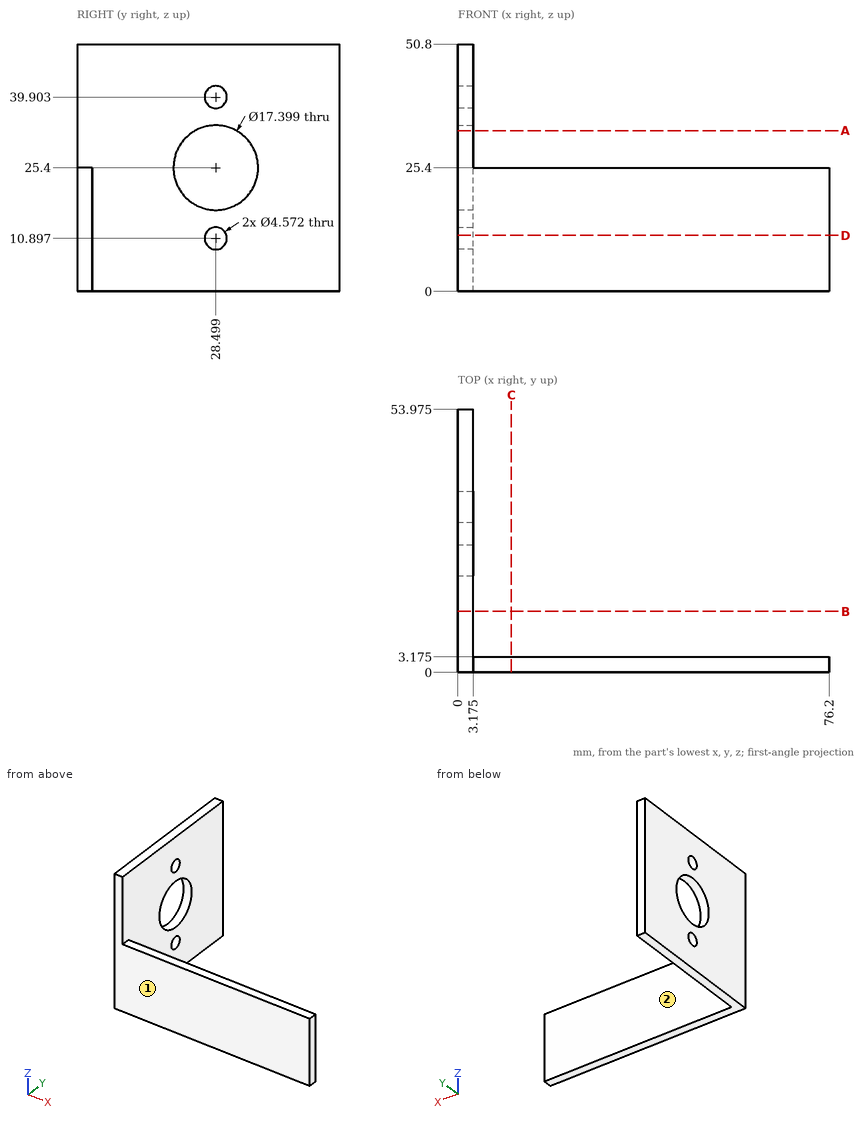
The drawing under review shows one solid part. Ordinate dimensions are in mm from its lowest x, y, z. A direction names the side the tool comes from. Coordinates: 2 decimals unless noted, no trailing zeros. Loops run counter-clockwise (first coordinate to the right, second up) from the corner with the lowest first, then second, coordinate; pieces in that order, holes last. Notation, with made-up numbers: (37.25, 64) - (55.25, 64) arc R12 ccw to (55.25, 80) - close; hole circle Ø1 at (46, -33.5). An arc over 180 degrees is marked (long way). Use CSV: the item, a comma, the result in double quotes. Start each with the question number.
1. To check wall thickness, follow probe 1 along Y at (x, z) = (0.85, 25.4) (1 decimal); probe 2 along X at (y, z) = (4, 5.5) (1 decimal). State the ranges of each line that lie inside material, in increasing order.
2. For the marked faces 1 and 2, list the 3-axis set-ups (+Z, -Z, +X, -X, +Y, -Y) from which the entire face can be reached by the end or side of a thin tool; tool diameter is ignored.
3. Add section B-B on y = 12.5. Give the boundary of the cut face in (x, z) (1 decimal).
4. Add section C-C on x = 11. Give the boundary of the cut face in (y, z) (1 decimal).
5. Add section D-D on z = 11.5. Give the boundary of the cut face in (x, y) (1 decimal), plus the area to 3 significant figures.
6. Clearance check with flat-ended pins moving along their axes: pin 1 (4 mm diameter, centred on y = 34.5, z = 42.5, fed in from +X) (3 decimals); pin 2 (1.6 mm diameter, centred on x = 39, y = 2, fed in from +Z); pin 3 (14 mm diameter, centred on y = 28.5, z = 25.4, fed in from -X); pin 4 (1 mm diameter, centred on x = 67.5, z = 25.5, fed in from +Y) (3 decimals). State where each tip first meets the part, or that it passes through.
7. Add section A-A on z = 33. Give the boundary of the cut face in (x, y) (1 decimal).
Resolved:
1,probe 1,"0 to 19.8, 37.2 to 54"
1,probe 2,"0 to 3.2"
2,face 1,"+Z, -Z, +X, -X, -Y"
2,face 2,"+Z, -Z, +X, +Y"
3,outline,"(0, 0) - (3.2, 0) - (3.2, 50.8) - (0, 50.8) - close"
4,outline,"(0, 0) - (3.2, 0) - (3.2, 25.4) - (0, 25.4) - close"
5,outline,"(0, 0) - (76.2, 0) - (76.2, 3.2) - (3.2, 3.2) - (3.2, 26.3) - (0, 26.3) - close; (0, 30.7) - (3.2, 30.7) - (3.2, 54) - (0, 54) - close"
5,area,"389 mm2"
6,pin 1,"x = 3.175"
6,pin 2,"z = 25.4"
6,pin 3,"through"
6,pin 4,"y = 3.175"
7,outline,"(0, 0) - (3.2, 0) - (3.2, 24.3) - (0, 24.3) - close; (0, 32.7) - (3.2, 32.7) - (3.2, 54) - (0, 54) - close"
